Study the drawing (mm; zero at the part's minimum x, y, z) and answer. A direction names the side the tool comes from. Round coordinates to 2 decimals unless told otherwise and drop trailing zeros. Loops run counter-clockwise (first coordinate to the right, second up) from the corner with the lowest first, then second, coordinate; pieces in that order, holes last. Notation, with made-up numbers: M 34,55.25 L 82,55.25 A7 ccw 82,67.25 Z; hole C -25.5,79.25 d10. An arc over 180 degrees is marked long. Write each question's results on one line, items separated by ' | '.
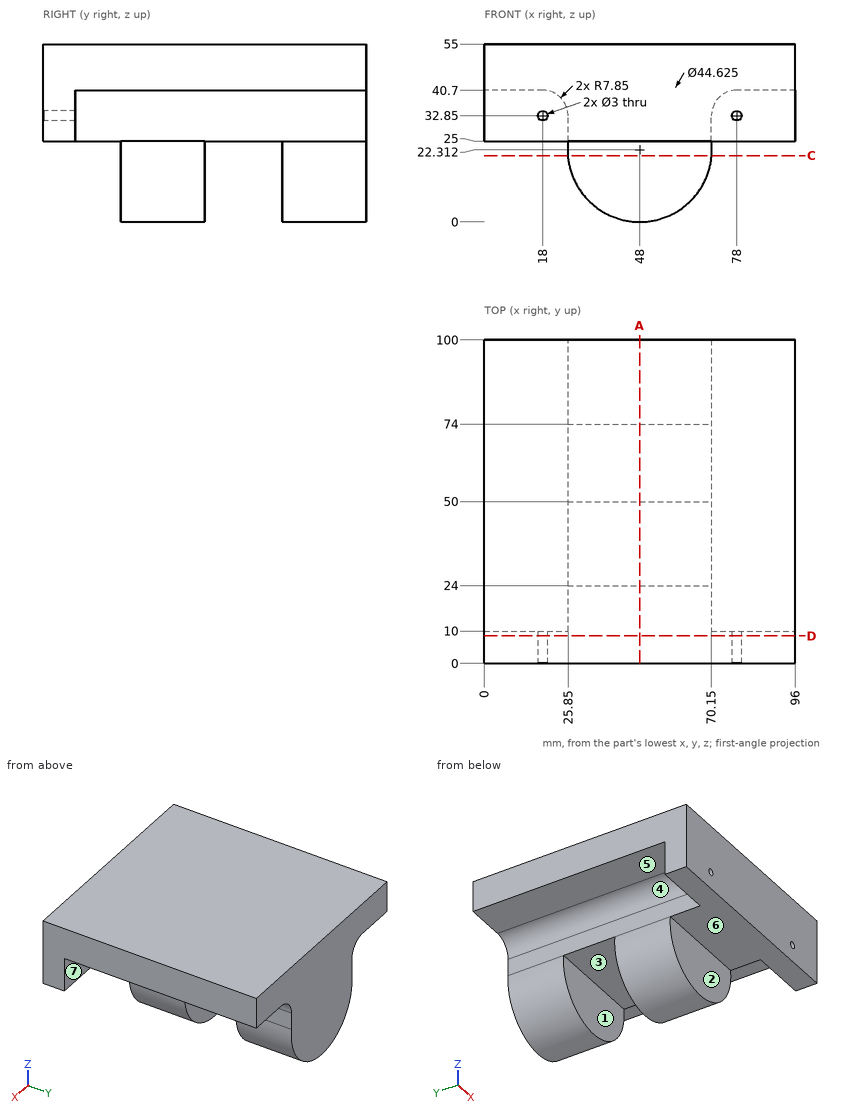
Item 1: Straight lines are drawn through the part: line 1 (Z direction, x = 18, y = 7.5); line 2 (X direction, y = 4, z = 32) (1 decimal); line 3 (Y direction, x = 55, z = 10). For each, find the intervals that lie inside material, in ascending order.
Outcome:
line 1: z = 25 to 31.35, 34.35 to 55 | line 2: x = 0 to 16.8, 19.2 to 76.8, 79.2 to 96 | line 3: y = 24 to 50, 74 to 100
Item 2: The mould has two halves that part along Y. Classify the marked faces 1, 2, 3 and 4: pulls with the +Y half, pulls with the -Y half, needs draft (parallel to the pull), parting line crosses it, or undercut.
Outcome:
face 1: undercut | face 2: pulls with the -Y half | face 3: undercut | face 4: needs draft
Item 3: The part is cut by section D-D (y = 8.5). Determine the outline of the cut face in (x, z), plus the area to 3 significant figures.
Outcome:
outline: M 0,25 L 96,25 L 96,55 L 0,55 Z; hole C 18,32.85 d3; hole C 78,32.85 d3 | area: 2,870 mm2
Item 4: The part is cut by section C-C (z = 20.5). Determine the outline of the cut face in (x, y), plus the area to 3 significant figures.
Outcome:
outline: M 25.76,24 L 70.24,24 L 70.24,50 L 25.76,50 Z; M 25.76,74 L 70.24,74 L 70.24,100 L 25.76,100 Z | area: 2,310 mm2
Item 5: For the marked faces 5, 6 and 7, determine the directions among +Z, -Z, +X, -X, +Y, -Y from which every point of the face is accessible in a straight line to the end or side of a thin tool.
Outcome:
face 5: -Z, -X, +Y | face 6: -Z, +X, -X, -Y | face 7: -Z, +X, +Y
Item 6: Flat-ended cylindrical pins translate along their axes: pin 1 (5 mm diameter, centred on x = 47.5, y = 77, fed in from -Z); pin 2 (12.5 mm diameter, centred on x = 12.5, z = 36.5, fed in from +Y); pin 3 (3.5 mm diameter, centred on x = 78, z = 32.85, fed in from +Y); pin 4 (3 mm diameter, centred on y = 15.5, z = 28, fed in from +X). Find the tip coordinate at first contact, or state that the pin passes through.
Outcome:
pin 1: stops at z = 0 | pin 2: stops at y = 100 | pin 3: stops at y = 10 | pin 4: stops at x = 70.15
Item 7: The part is cut by section A-A (x = 48). Determine the outline of the cut face in (y, z), plus the area to 3 significant figures.
Outcome:
outline: M 0,25 L 24,25 L 24,0 L 50,0 L 50,25 L 74,25 L 74,0 L 100,0 L 100,55 L 0,55 Z | area: 4,300 mm2
